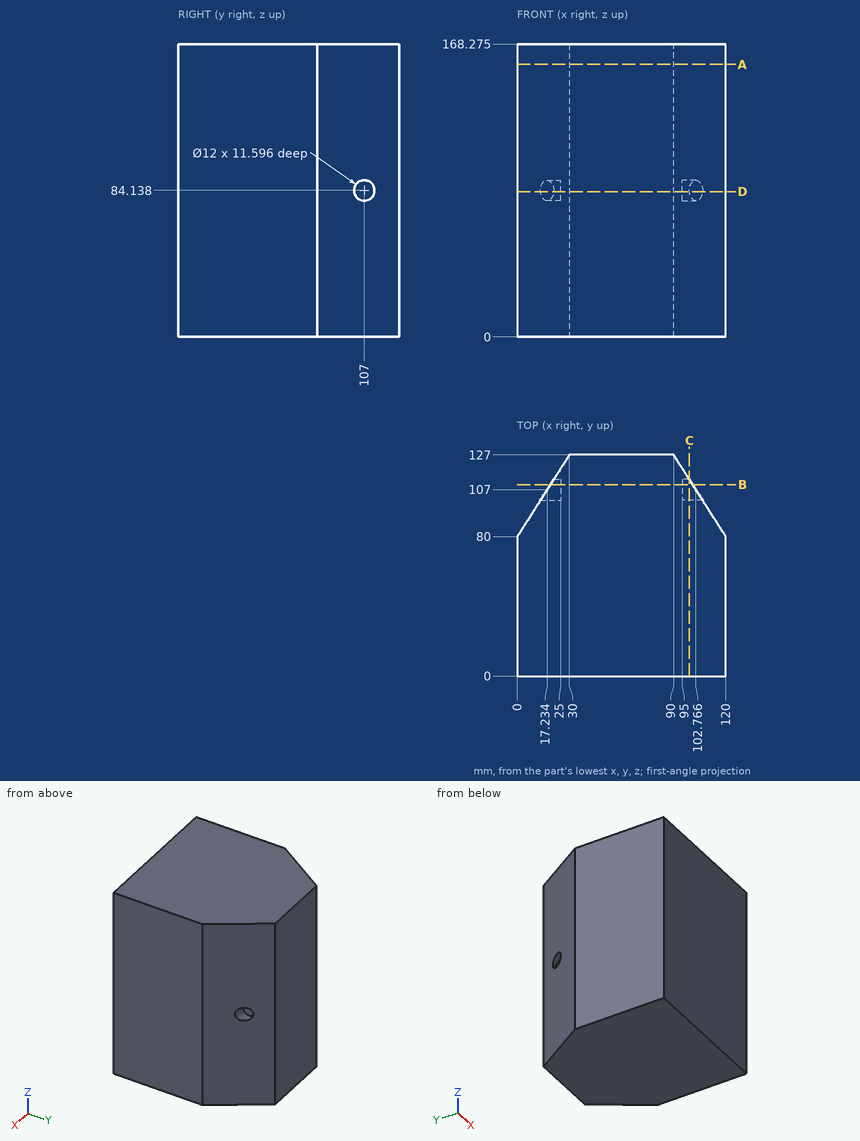
Here's the drawing with two shaded views (mm, measured from the low corner). I have some questions. Round coordinates to 2 decimals unless told otherwise and drop trailing zeros. Order: outer loops, then holes, each group sorted by start corner. A loop starts at its lowest first (then second) coordinate and runs counter-clockwise, first axis right, second up. Notation, with made-up numbers: (15.25, 42) -> (45.25, 42) arc R17 cw to (45.25, 65) -> close; hole circle Ø11 at (-4, 81.5). An arc over 180 degrees is marked (long way). Use a Markdown table: item, result. Add a question column.
(1) Suppose I cut it at C-C, the plane x = 99. Please give me the cut outline in (y, z) (1 decimal).
(2) Suppose I cut it at D-D, the plane z = 83.5. Please give me the cut outline in (x, y) (1 decimal), and give its area (3 significant figures).
(3) For pin 1 Ø7 at (y, z) = (107, 84.14) entering from +X; pin 2 Ø1.5 at (x, z) = (26, 126) entering from +Y; pin 3 Ø14 at (y, z) = (107, 84.14) entering from -X (1 decimal), each with a flat end and sliding along its axis, tell me the tip position at first contact or that it passes through.
(4) Suppose I cut it at A-A, the plane z = 156.5. Please give me the cut outline in (x, y).
(5) Suppose I cut it at B-B, the plane y = 110. Please give me the cut outline in (x, z) (1 decimal).
(6) I need wall thicknesses on line 1 along Z through (x, y) = (99, 107) (1 decimal); line 2 along Y through (x, z) = (26.5, 146) (1 decimal); line 3 along X through (y, z) = (91, 15.5). Which ranges of each line are inside material? Lowest first, please.
Verdict:
| question | item | result |
|---|---|---|
| 1 | outline | (0, 0) -> (112.9, 0) -> (112.9, 83) arc R6 cw (long way) to (112.9, 85.2) -> (112.9, 168.3) -> (0, 168.3) -> close |
| 2 | outline | (0, 0) -> (120, 0) -> (120, 80) -> (106.6, 101) -> (95, 101) -> (95, 113) -> (99, 113) -> (90, 127) -> (30, 127) -> (21, 113) -> (25, 113) -> (25, 101) -> (13.4, 101) -> (0, 80) -> close |
| 2 | area | 13,600 mm2 |
| 3 | pin 1 | x = 95 |
| 3 | pin 2 | y = 121.91 |
| 3 | pin 3 | x = 12.8 |
| 4 | outline | (0, 0) -> (120, 0) -> (120, 80) -> (90, 127) -> (30, 127) -> (0, 80) -> close |
| 5 | outline | (19.1, 0) -> (100.9, 0) -> (100.9, 78.9) -> (95, 78.9) -> (95, 89.3) -> (100.9, 89.3) -> (100.9, 168.3) -> (19.1, 168.3) -> (19.1, 89.3) -> (25, 89.3) -> (25, 78.9) -> (19.1, 78.9) -> close |
| 6 | line 1 | 0 to 78.1, 90.1 to 168.3 |
| 6 | line 2 | 0 to 121.5 |
| 6 | line 3 | 7.02 to 112.98 |
